```python
from build123d import *

# Parameters (mm, degrees)
BASPROSKE_W     = 2
BASPROSKE_H     = 4.5
TOOTHCUT_DEPTH  = 7.670832032
TEETHCUTS_COUNT = 16
TEETHCUTS_ANGLE = 337.5
BORSKE_R        = 1.65
BORE_DEPTH      = 50.0000508
EXTRUDE_2_DEPTH = 0.3
FILLET_4_R      = 0.1
FILLET_5_R      = 0.1
FILLET_6_R      = 0.1
EXTRUDE_START   = -2.3
EXTRUDE_5_DEPTH = 0.3
FILLET_7_R      = 0.1
FILLET_8_R      = 0.1
FILLET_9_R      = 0.1


with BuildPart() as part:
    # BasProSke → Base-Revolve (revolve)
    with BuildSketch(Plane(origin=(0, 0, 0), x_dir=(1, 0, 0), z_dir=(0, 1, 0)), mode=Mode.PRIVATE) as base_revolve_sk:
        with Locations((1, 2.25)):
            Rectangle(BASPROSKE_W, BASPROSKE_H)
    revolve(base_revolve_sk.sketch.rotate(Axis((-10, 0, 0), (1, 0, 0)), 180), axis=Axis((-10, 0, 0), (1, 0, 0)))

    # TooCutSke → ToothCut (cut, through all)
    with BuildSketch(Plane(origin=(0, 0, 0), x_dir=(0, 0, -1), z_dir=(1, 0, 0))):
        with BuildLine():
            ThreePointArc((0.306025637, 3.360092902), (0, 3.374), (-0.306025637, 3.360092902))
            ThreePointArc((-0.306025637, 3.360092902), (-0.415941512, 3.953968919), (-0.738171669, 4.464789776))
            ThreePointArc((-0.738171669, 4.464789776), (0, 4.5254), (0.738171669, 4.464789776))
            ThreePointArc((0.738171669, 4.464789776), (0.415941512, 3.953968919), (0.306025637, 3.360092902))
        make_face()
    toothcut = extrude(amount=TOOTHCUT_DEPTH, mode=Mode.SUBTRACT)

    # TeethCuts: ToothCut ×16 about axis
    teethcuts_axis = Axis((-10, 0, 0), (1, 0, 0))
    for i in range(1, TEETHCUTS_COUNT):
        add(toothcut.rotate(teethcuts_axis, i * TEETHCUTS_ANGLE / (TEETHCUTS_COUNT - 1)), mode=Mode.SUBTRACT)

    # BorSke → Bore (cut, symmetric)
    with BuildSketch(Plane(origin=(0, 0, 0), x_dir=(0, 0, -1), z_dir=(1, 0, 0))):
        with Locations(Location((0, 0, 0), (0, 0, 180))):
            Circle(BORSKE_R)
    extrude(amount=BORE_DEPTH, both=True, mode=Mode.SUBTRACT)

    # 草图1 → 拉伸-薄壁2 (add)
    with BuildSketch(Plane(origin=(2, 0, 0), x_dir=(0, 0, -1), z_dir=(1, 0, 0))):
        with BuildLine():
            ThreePointArc((-1.1, 1.905255888), (0, 2.2), (1.1, 1.905255888))
            Line((1.1, 1.905255888), (1.2, 2.078460969))
            ThreePointArc((1.2, 2.078460969), (0, 2.4), (-1.2, 2.078460969))
            Line((-1.2, 2.078460969), (-1.1, 1.905255888))
        make_face()
        with BuildLine():
            ThreePointArc((2.2, 0), (1.905255888, -1.1), (1.1, -1.905255888))
            Line((1.1, -1.905255888), (1.2, -2.078460969))
            ThreePointArc((1.2, -2.078460969), (2.078460969, -1.2), (2.4, 0))
            Line((2.4, 0), (2.2, 0))
        make_face()
        with BuildLine():
            ThreePointArc((-1.1, -1.905255888), (-1.905255888, -1.1), (-2.2, 0))
            Line((-2.2, 0), (-2.4, 0))
            ThreePointArc((-2.4, 0), (-2.078460969, -1.2), (-1.2, -2.078460969))
            Line((-1.2, -2.078460969), (-1.1, -1.905255888))
        make_face()
    extrude(amount=EXTRUDE_2_DEPTH)

    # 圆角4
    # the kernel refuses this fillet: 0.1 mm, written as the material it takes off along each edge
    with BuildSketch(Plane(origin=(2.3, 0, 0), x_dir=(0, 0.10399688261682524, 0.994577623117463), z_dir=(0, 0.994577623117463, -0.10399688261682524))) as fillet_4_piece_1:
        with BuildLine():
            CenterArc((2.4 - FILLET_4_R, -FILLET_4_R), FILLET_4_R, 0, 90)
            Line((2.4 - FILLET_4_R, 0), (2.4, 0))
            Line((2.4, 0), (2.4, -FILLET_4_R))
        make_face()
    revolve(axis=Axis((2.3, 0, 0), (1, 0, 0)), revolution_arc=71.938751527, mode=Mode.SUBTRACT)
    with BuildSketch(Plane(origin=(2.3, 0, 0), x_dir=(0, -0.9171438900620574, 0.39855625063701683), z_dir=(0, -0.39855625063701683, -0.9171438900620574))) as fillet_4_piece_2:
        with BuildLine():
            CenterArc((2.2 + FILLET_4_R, FILLET_4_R), FILLET_4_R, 180, 90)
            Line((2.2 + FILLET_4_R, 0), (2.2, 0))
            Line((2.2, 0), (2.2, FILLET_4_R))
        make_face()
    revolve(axis=Axis((2.3, 0, 0), (-1, 0, 0)), revolution_arc=73.024092575, mode=Mode.SUBTRACT)

    # 圆角5
    # the kernel refuses this fillet: 0.1 mm, written as the material it takes off along each edge
    with BuildSketch(Plane(origin=(2.3, 0, 0), x_dir=(0, 0.809331046346937, -0.5873527538191783), z_dir=(0, -0.5873527538191783, -0.809331046346937))) as fillet_5_piece_1:
        with BuildLine():
            CenterArc((2.4 - FILLET_5_R, -FILLET_5_R), FILLET_5_R, 0, 90)
            Line((2.4 - FILLET_5_R, 0), (2.4, 0))
            Line((2.4, 0), (2.4, -FILLET_5_R))
        make_face()
    revolve(axis=Axis((2.3, 0, 0), (1, 0, 0)), revolution_arc=71.938751527, mode=Mode.SUBTRACT)
    with BuildSketch(Plane(origin=(2.3, 0, 0), x_dir=(0, 0.8037317829196821, 0.5949917824010252), z_dir=(0, -0.5949917824010252, 0.8037317829196821))) as fillet_5_piece_2:
        with BuildLine():
            CenterArc((2.2 + FILLET_5_R, FILLET_5_R), FILLET_5_R, 180, 90)
            Line((2.2 + FILLET_5_R, 0), (2.2, 0))
            Line((2.2, 0), (2.2, FILLET_5_R))
        make_face()
    revolve(axis=Axis((2.3, 0, 0), (-1, 0, 0)), revolution_arc=73.024092575, mode=Mode.SUBTRACT)

    # 圆角6
    # the kernel refuses this fillet: 0.1 mm, written as the material it takes off along each edge
    with BuildSketch(Plane(origin=(2.3, 0, 0), x_dir=(0, -0.9133279289636526, -0.4072248692982359), z_dir=(0, -0.4072248692982359, 0.9133279289636526))) as fillet_6_piece_1:
        with BuildLine():
            CenterArc((2.4 - FILLET_6_R, -FILLET_6_R), FILLET_6_R, 0, 90)
            Line((2.4 - FILLET_6_R, 0), (2.4, 0))
            Line((2.4, 0), (2.4, -FILLET_6_R))
        make_face()
    revolve(axis=Axis((2.3, 0, 0), (1, 0, 0)), revolution_arc=71.938751527, mode=Mode.SUBTRACT)
    with BuildSketch(Plane(origin=(2.3, 0, 0), x_dir=(0, 0.11341210714236213, -0.9935480330379249), z_dir=(0, 0.9935480330379249, 0.11341210714236213))) as fillet_6_piece_2:
        with BuildLine():
            CenterArc((2.2 + FILLET_6_R, FILLET_6_R), FILLET_6_R, 180, 90)
            Line((2.2 + FILLET_6_R, 0), (2.2, 0))
            Line((2.2, 0), (2.2, FILLET_6_R))
        make_face()
    revolve(axis=Axis((2.3, 0, 0), (-1, 0, 0)), revolution_arc=73.024092575, mode=Mode.SUBTRACT)

    # 草图1<5> → 拉伸-薄壁5 (add)
    with BuildSketch(Plane(origin=(2, 0, 0), x_dir=(0, 0, -1), z_dir=(1, 0, 0)).offset(EXTRUDE_START)):
        with BuildLine():
            ThreePointArc((-1.1, 1.905255888), (0, 2.2), (1.1, 1.905255888))
            Line((1.1, 1.905255888), (1.2, 2.078460969))
            ThreePointArc((1.2, 2.078460969), (0, 2.4), (-1.2, 2.078460969))
            Line((-1.2, 2.078460969), (-1.1, 1.905255888))
        make_face()
        with BuildLine():
            ThreePointArc((2.2, 0), (1.905255888, -1.1), (1.1, -1.905255888))
            Line((1.1, -1.905255888), (1.2, -2.078460969))
            ThreePointArc((1.2, -2.078460969), (2.078460969, -1.2), (2.4, 0))
            Line((2.4, 0), (2.2, 0))
        make_face()
        with BuildLine():
            ThreePointArc((-1.1, -1.905255888), (-1.905255888, -1.1), (-2.2, 0))
            Line((-2.2, 0), (-2.4, 0))
            ThreePointArc((-2.4, 0), (-2.078460969, -1.2), (-1.2, -2.078460969))
            Line((-1.2, -2.078460969), (-1.1, -1.905255888))
        make_face()
    extrude(amount=EXTRUDE_5_DEPTH)

    # 圆角7
    # the kernel refuses this fillet: 0.1 mm, written as the material it takes off along each edge
    with BuildSketch(Plane(origin=(-0.3, 0, 0), x_dir=(0, 0.809331046346937, -0.5873527538191783), z_dir=(0, -0.5873527538191783, -0.809331046346937))) as fillet_7_piece_1:
        with BuildLine():
            CenterArc((2.4 - FILLET_7_R, FILLET_7_R), FILLET_7_R, 270, 90)
            Line((2.4 - FILLET_7_R, 0), (2.4, 0))
            Line((2.4, 0), (2.4, FILLET_7_R))
        make_face()
    revolve(axis=Axis((-0.3, 0, 0), (1, 0, 0)), revolution_arc=71.938751527, mode=Mode.SUBTRACT)
    with BuildSketch(Plane(origin=(-0.3, 0, 0), x_dir=(0, 0.8037317829196821, 0.5949917824010252), z_dir=(0, -0.5949917824010252, 0.8037317829196821))) as fillet_7_piece_2:
        with BuildLine():
            CenterArc((2.2 + FILLET_7_R, -FILLET_7_R), FILLET_7_R, 90, 90)
            Line((2.2 + FILLET_7_R, 0), (2.2, 0))
            Line((2.2, 0), (2.2, -FILLET_7_R))
        make_face()
    revolve(axis=Axis((-0.3, 0, 0), (-1, 0, 0)), revolution_arc=73.024092575, mode=Mode.SUBTRACT)

    # 圆角8
    # the kernel refuses this fillet: 0.1 mm, written as the material it takes off along each edge
    with BuildSketch(Plane(origin=(-0.3, 0, 0), x_dir=(0, 0.10399688261682512, 0.994577623117463), z_dir=(0, 0.994577623117463, -0.10399688261682512))) as fillet_8_piece_1:
        with BuildLine():
            CenterArc((2.4 - FILLET_8_R, FILLET_8_R), FILLET_8_R, 270, 90)
            Line((2.4 - FILLET_8_R, 0), (2.4, 0))
            Line((2.4, 0), (2.4, FILLET_8_R))
        make_face()
    revolve(axis=Axis((-0.3, 0, 0), (1, 0, 0)), revolution_arc=71.938751527, mode=Mode.SUBTRACT)
    with BuildSketch(Plane(origin=(-0.3, 0, 0), x_dir=(0, -0.9171438900620574, 0.39855625063701694), z_dir=(0, -0.39855625063701694, -0.9171438900620574))) as fillet_8_piece_2:
        with BuildLine():
            CenterArc((2.2 + FILLET_8_R, -FILLET_8_R), FILLET_8_R, 90, 90)
            Line((2.2 + FILLET_8_R, 0), (2.2, 0))
            Line((2.2, 0), (2.2, -FILLET_8_R))
        make_face()
    revolve(axis=Axis((-0.3, 0, 0), (-1, 0, 0)), revolution_arc=73.024092575, mode=Mode.SUBTRACT)

    # 圆角9
    # the kernel refuses this fillet: 0.1 mm, written as the material it takes off along each edge
    with BuildSketch(Plane(origin=(-0.3, 0, 0), x_dir=(0, -0.9133279289636526, -0.4072248692982359), z_dir=(0, -0.4072248692982359, 0.9133279289636526))) as fillet_9_piece_1:
        with BuildLine():
            CenterArc((2.4 - FILLET_9_R, FILLET_9_R), FILLET_9_R, 270, 90)
            Line((2.4 - FILLET_9_R, 0), (2.4, 0))
            Line((2.4, 0), (2.4, FILLET_9_R))
        make_face()
    revolve(axis=Axis((-0.3, 0, 0), (1, 0, 0)), revolution_arc=71.938751527, mode=Mode.SUBTRACT)
    with BuildSketch(Plane(origin=(-0.3, 0, 0), x_dir=(0, 0.11341210714236213, -0.9935480330379249), z_dir=(0, 0.9935480330379249, 0.11341210714236213))) as fillet_9_piece_2:
        with BuildLine():
            CenterArc((2.2 + FILLET_9_R, -FILLET_9_R), FILLET_9_R, 90, 90)
            Line((2.2 + FILLET_9_R, 0), (2.2, 0))
            Line((2.2, 0), (2.2, -FILLET_9_R))
        make_face()
    revolve(axis=Axis((-0.3, 0, 0), (-1, 0, 0)), revolution_arc=73.024092575, mode=Mode.SUBTRACT)


solid = part.part
```
Input: part model. Units: mm. Frame: model coordinates. A direction names the side the tool comes from. Round coordinates to 2 decimals unless told otherwise and drop trailing zeros. Loops run counter-clockwise (first coordinate to the right, second up) from the corner with the lowest first, then second, coordinate; pieces in that order, holes last. Notation, with made-up numbers: (2.25, 30.25) - (42.25, 30.25) arc R10 ccw to (42.25, 36.25) - close; hole circle Ø10 at (75.25, 70.25). An arc over 180 degrees is marked (long way). One line per item, written item: value. Start each with the question number.
(1) Section A-A, the plane z = 0. Return loops of the section in (x, y).
(2) Section C-C, the plane y = 0.5. Return loops of the section in (x, z), plus the area to 3 significant figures.
(3) Ray query, line 1 (Y direction, x = 1.1, z = 0); line 2 (Y direction, x = 1.65, z = 2.5); line 3 (Z direction, x = 0.95, y = -3.5). Return the intervals inside material, ascending. Write a range as [from, to].
(4) Draft query along Z for faces 3 (the cylindrical face through (0.99, -3.79, 1.13)), 4 (the cylindrical face through (0.986, -1.881, 3.477)). Return one class per face: +Z half, -Z half, draft (parallel to the pull), parting line (faces both ways), or undercut.
(5) Access query for faces 1 (the cylindrical face through (0.99, -3.81, -1.13)), 2 (the cylindrical face through (0.986, -3.477, -1.881)). Directions: +Z, -Z, +X, -X, +Y, -Y. A direction counts if a zero-diameter tool reaches every point of the face in a straight line with its end or side. Return the directions, or none.
(6) Section B-B, the plane y = -3.5. Return loops of the section in (x, z), plus the area to 3 significant figures.
(7) Contact query for flat-ended pins moving along their axis: P1, Ø1.5, axis at x = 1.5, z = 2, coming from the +Y side; P2, Ø1.5, axis at y = 1.5, z = 3, coming from the +X side. Output: stop coordinate, or through.
Results below:
1. outline: (-0.2, 2.2) - (0, 2.2) - (0, 1.65) - (2, 1.65) - (2, 2.2) - (2.2, 2.2) arc R0.1 ccw to (2.2, 2.4) - (2, 2.4) - (2, 3.37) - (0, 3.37) - (0, 2.4) - (-0.2, 2.4) arc R0.1 ccw to start; (0, -3.37) - (2, -3.37) - (2, -1.65) - (0, -1.65) - close
2. outline: (0, -4.13) - (2, -4.13) - (2, -1.57) - (0, -1.57) - close; (0, 1.57) - (2, 1.57) - (2, 4.13) - (0, 4.13) - close
2. area: 10.2 mm^2
3. line 1: [-3.37, -1.65], [1.65, 3.37]
3. line 2: [-3.74, -3.09], [-2.27, 2.27], [3.09, 3.74]
3. line 3: [-2.62, -1.9], [-1.09, -0.31], [0.31, 1.09], [1.9, 2.62]
4. face 3: undercut
4. face 4: +Z half
5. face 1: +X, -X
5. face 2: +X, -X, -Y
6. outline: (0, -2.62) - (2, -2.62) - (2, -1.9) - (0, -1.9) - close; (0, -1.09) - (2, -1.09) - (2, -0.31) - (0, -0.31) - close; (0, 0.31) - (2, 0.31) - (2, 1.09) - (0, 1.09) - close; (0, 1.9) - (2, 1.9) - (2, 2.62) - (0, 2.62) - close
6. area: 5.99 mm^2
7. P1: y = 3.83
7. P2: x = 2
